```python
from build123d import *

# Parameters (mm, degrees)
F0_R     = 50
F0_R_2   = 37.5
F1_DEPTH = 15
F2_W     = 110
F2_H     = 64.89666
F3_DEPTH = 15.001
F4_R     = 3
F5_DEPTH = 50.001
F7_R     = 5.5
F8_DEPTH = 25


with BuildPart() as f1:
    # F0 (on Top) → F1 (new body)
    with BuildSketch(Plane.XY):
        Circle(F0_R)
        Circle(F0_R_2, mode=Mode.SUBTRACT)
    extrude(amount=F1_DEPTH)

    # F2 (on face) → F3 (cut, through all)
    with BuildSketch(Plane.XY.offset(15)):
        with Locations((0, -30.94833)):
            Rectangle(F2_W, F2_H)
    extrude(amount=-F3_DEPTH, mode=Mode.SUBTRACT)

    # F4 (on Front) → F5 (cut, through all)
    with BuildSketch(Plane.XZ):
        with Locations((-43.723741, 7.5)):
            Circle(F4_R)
        with Locations((43.723741, 7.5)):
            Circle(F4_R)
    extrude(amount=-F5_DEPTH, mode=Mode.SUBTRACT)

    # F7 (on offset) → F8 (cut)
    with BuildSketch(Plane.XZ.offset(-10)):
        with Locations((43.723741, 7.5)):
            Circle(F7_R)
        with Locations((-43.723741, 7.5)):
            Circle(F7_R)
    extrude(amount=-F8_DEPTH, mode=Mode.SUBTRACT)


solid = f1.part
```
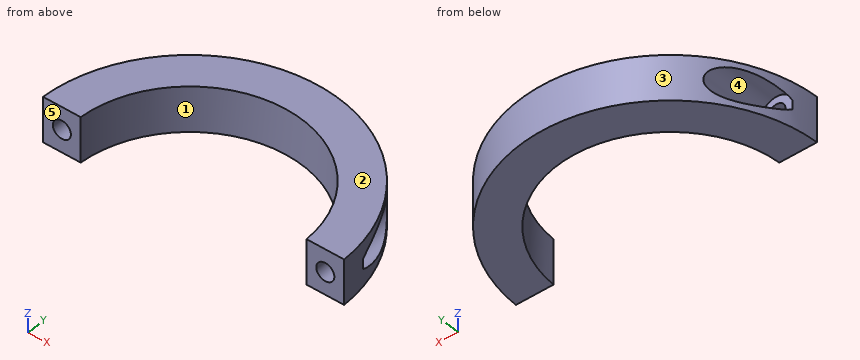
Model file for the job. Use its own axes, mm. Face numbers are marked on the shaded views. A direction names the side the tool comes from. Give positions to 0.01 mm unless a question says otherwise; leave off trailing zeros. Loops run counter-clockwise (first coordinate to the right, second up) from the corner with the lowest first, then second, coordinate; pieces in that order, holes last. Notation, with made-up numbers: (9, 33.25) - (29, 33.25) arc R27 cw to (29, 72.25) - close; hole circle Ø10 at (22, -31.5). An arc over 180 degrees is marked (long way). One line per item, written item: value. Start each with the question number.
1. Slice it at B-B (y = 15). List the corners of the cut face in (x, z), plus the area to 3 significant figures.
2. Probe L1, parallel to X at y = 5.5, z = 8.5; L2, parallel to Z at x = -44.5, y = 13; L3, parallel to X at y = 28.5, z = 1. List the from-to ranges inside material, lowest first. Write a range as from..to.
3. Pin check, flat tips, straight feed: pin 1 (2 mm diameter, centred on x = 22, z = 4, fed in from -Y); pin 2 (5.5 mm diameter, centred on x = 41.5, z = 6.5, fed in from +Y); pin 3 (3 mm diameter, centred on x = -16.5, z = 13, fed in from -Y). Stop position of each tip, or through.
4. Slice it at D-D (z = 3.25). List the corners of the cut face in (x, y), plus the area to 3 significant figures.
5. Which spindle directions (+Z, -Z, +X, -X, +Y, -Y) get a long thin tool onto all of the face, cutting with end or side? Do the marked faces 4 and 5. Say none if no direction does.
6. Slice it at A-A (z = 7.5). List the corners of the cut face in (x, y), plus the area to 3 significant figures.
7. Slice it at C-C (x = 43.5). List the corners of the cut face in (y, z), plus the area to 3 significant figures.
8. Pull direction X, two halves, no side cores. Call the marked faces 1, 2 and 3: pulls with the +X half, pulls with the -X half, needs draft (parallel to the pull), parting line crosses it, or undercut.
Solution:
1. outline: (-47.7, 0) - (-34.37, 0) - (-34.37, 15) - (-47.7, 15) - (-47.7, 11.3) arc R5.5 cw (long way) to (-47.7, 3.7) - close; (34.37, 0) - (47.7, 0) - (47.7, 3.7) arc R5.5 cw (long way) to (47.7, 11.3) - (47.7, 15) - (34.37, 15) - close
1. area: 226 mm^2
2. L1: x = -49.7..-46.55, -40.9..-37.09, 37.09..40.9, 46.55..49.7
2. L2: z = 0..2.06, 12.94..15
2. L3: x = -41.08..-24.37, 24.37..41.08
3. pin 1: stops at y = 29.62
3. pin 2: stops at y = 10
3. pin 3: stops at y = 32.9
4. outline: (-49.98, 1.5) - (-37.47, 1.5) arc R37.5 cw to (37.47, 1.5) - (49.98, 1.5) arc R50 ccw to (47.21, 16.45) - (47.21, 10) - (40.23, 10) - (40.23, 29.69) arc R50 ccw to (-40.23, 29.69) - (-40.23, 10) - (-47.21, 10) - (-47.21, 16.45) arc R50 ccw to start
4. area: 1,490 mm^2
5. face 4: +Y
5. face 5: +Z, -Z, +X, -X, -Y
6. outline: (-49.98, 1.5) - (-46.72, 1.5) - (-46.72, 10) - (-48.99, 10) arc R50 ccw to start; (-40.72, 1.5) - (-37.47, 1.5) arc R37.5 cw to (37.47, 1.5) - (40.72, 1.5) - (40.72, 10) - (38.22, 10) - (38.22, 32.23) arc R50 ccw to (-38.22, 32.23) - (-38.22, 10) - (-40.72, 10) - close; (46.72, 1.5) - (49.98, 1.5) arc R50 ccw to (48.99, 10) - (46.72, 10) - close
6. area: 1,290 mm^2
7. outline: (1.5, 0) - (24.65, 0) - (24.65, 2) - (10, 2) - (10, 4.51) - (1.5, 4.51) - close; (1.5, 10.49) - (10, 10.49) - (10, 13) - (24.65, 13) - (24.65, 15) - (1.5, 15) - close
7. area: 135 mm^2
8. face 1: undercut
8. face 2: needs draft
8. face 3: parting line crosses it
